from build123d import *

# Parameters (mm, degrees)
ESQUISSE2_R             = 10.125
BOSS_EXTRU_1_DEPTH      = 10
ENL_V_MAT_EXTRU_1_DEPTH = 218.649228582
BOSS_EXTRU_2_START      = -3.3
BOSS_EXTRU_2_DEPTH      = 3.3


with BuildPart() as part:
    # Esquisse1 → Révolution1 (revolve)
    with BuildSketch(Plane(origin=(0, 72.395438751, 0), x_dir=(-1, 0, 0), z_dir=(0, 1, 0))):
        Polygon((91.397628985, 206.017597396), (92.357726425, 191.749864118), (95.650280259, 191.971425065), (94.690182819, 206.239158344), align=None)
    revolve(axis=Axis((-92.670542197, 72.395438751, 191.770913966), (-0.9977435859079083, 0, 0.06713968111056465)))

    # Esquisse2 → Boss.-Extru.1 (add)
    with BuildSketch(Plane(origin=(-108.078931537, 0, 7.272795436), x_dir=(0.06713968111057397, 0, 0.9977435859079078), z_dir=(-0.9977435859079079, 0, 0.06713968111057397))):
        with Locations((185.116328722, 72.395438751)):
            Circle(ESQUISSE2_R)
    extrude(amount=BOSS_EXTRU_1_DEPTH)

    # Esquisse3 → Enlèv. mat.-Extru.1 (cut, through all)
    with BuildSketch(Plane(origin=(-104.786377704, 0, 7.051234489), x_dir=(-0.06713968111057397, 0, -0.9977435859079078), z_dir=(0.9977435859079079, 0, -0.06713968111057397))):
        with BuildLine():
            Line((-186.241328722, 77.751028507), (-186.241328722, 79.051028507))
            ThreePointArc((-186.241328722, 79.051028507), (-185.116328722, 65.645438751), (-183.991328722, 79.051028507))
            Line((-183.991328722, 79.051028507), (-183.991328722, 77.751028507))
            Line((-183.991328722, 77.751028507), (-186.241328722, 77.751028507))
        make_face()
    extrude(amount=-ENL_V_MAT_EXTRU_1_DEPTH, mode=Mode.SUBTRACT)

    # Esquisse8 → Boss.-Extru.2 (add)
    with BuildSketch(Plane(origin=(-108.078931537, 0, 7.272795436), x_dir=(0.06713968111056465, 0, 0.9977435859079083), z_dir=(-0.9977435859079085, 0, 0.06713968111056466)).offset(BOSS_EXTRU_2_START)):
        with BuildLine():
            Line((181.116328722, 58.666272717), (181.116328722, 51.895438751))
            Line((181.116328722, 51.895438751), (189.116328722, 51.895438751))
            Line((189.116328722, 51.895438751), (189.116328722, 58.666272717))
            ThreePointArc((189.116328722, 58.666272717), (185.116328722, 58.095438751), (181.116328722, 58.666272717))
        make_face()
    extrude(amount=BOSS_EXTRU_2_DEPTH)


solid = part.part
Verification items for the finished model (mm, model axes). A direction names the side the tool comes from. Round coordinates to 2 decimals unless told otherwise and drop trailing zeros. Loops run counter-clockwise (first coordinate to the right, second up) from the corner with the lowest first, then second, coordinate; pieces in that order, holes last. Notation, with made-up numbers: M 3,54 L 40,54 A30 ccw 40,85 Z; hole C -23,18 d7. An arc over 180 degrees is marked long. Write each question's results on one line, items separated by ' | '.
1) Section check A-A on y = 74.5. Record the boundary of the cut face in (x, z).
Checks:
outline: M -106.29,182.76 L -96.32,182.09 L -96.6,177.86 L -93.31,177.64 L -92.79,185.35 L -106.06,186.24 Z; M -105.2,199.04 L -91.93,198.15 L -91.41,205.86 L -94.7,206.08 L -94.99,201.85 L -104.96,202.52 Z
2) Section check B-B on y = 71. Record the boundary of the cut face in (x, z).
Checks:
outline: M -106.3,182.64 L -96.32,181.97 L -96.61,177.77 L -93.31,177.55 L -92.8,185.16 L -106.07,186.05 Z; M -105.18,199.23 L -91.91,198.34 L -91.4,205.95 L -94.69,206.17 L -94.98,201.98 L -104.95,202.65 Z
3) Mould release check, pull along Y, two halves, no side actions. Record for faces 4 (the flat face through (-94, 51.895, 192)), 5 (the cylindrical face through (-93.943, 86.684, 192.43)), 6 (the flat face through (-98.975, 78.41, 191.068)), 7 (the flat face through (-93.71, 55.23, 195.85)): released by +Y, released by -Y, zero draft, split by the parting line, or undercut.
Checks:
face 4: released by -Y | face 5: split by the parting line | face 6: undercut | face 7: zero draft
4) Scan lines: L1, parallel to Y at x = -98.5, z = 196.25; L2, parallel to Y at x = -101.5, z = 198; L3, parallel to Z at x = -101.75, y = 74.5. Record each from-to range of solid material in increasing order. Write a range as from..to.
Checks:
L1: y = 63.13..67.02, 77.77..81.66 | L2: y = 63.97..68.66, 76.13..80.82 | L3: z = 182.46..185.95, 198.81..202.31
5) Section check D-D on y = 63.5. Record the boundary of the cut face in (x, z).
Checks:
outline: M -105.95,187.82 L -95.97,187.15 L -96.4,180.8 L -93.11,180.58 L -91.61,202.92 L -94.9,203.14 L -95.33,196.8 L -105.3,197.47 Z
6) Access from +Z, -Z, +X, -X, +Y, -Y to the whole of each face (thin tool, end or side, straight path). Record for faces 1 (the flat face through (-94.25, 55.33, 187.87)), 2 (the flat face through (-99, 77.751, 192)), 3 (the cylindrical face through (-100.26, 63.41, 196.96)).
Checks:
face 1: -Z, -X, -Y | face 2: +X, -X | face 3: none
7) Gauge pin test, flat ends, axial feed: P1, Ø8, axis at y = 76, z = 202, coming from the -X side; P2, Ø3, axis at x = -103, z = 195, coming from the +Y side; P3, Ø2.5, axis at x = -99, z = 192.5, coming from the -Y side. Record the tip position at first contact, or that the pin passes through.
Checks:
P1: stops at x = -105.27 | P2: stops at y = 82.47 | P3: stops at y = 62.27
8) Section check C-C on y = 79.5. Record the boundary of the cut face in (x, z).
Checks:
outline: M -106.11,185.45 L -96.13,184.77 L -96.48,179.59 L -93.19,179.37 L -91.52,204.13 L -94.82,204.35 L -95.17,199.17 L -105.14,199.84 Z
